from build123d import *

# Parameters (mm, degrees)
CUT_EXTRUDE_START   = 40
CUT_EXTRUDE_1_DEPTH = 15
SKETCH_3_R          = 2.5
EXTRUDE_1_DEPTH     = 3
FILLET_1_R          = 1


with BuildPart() as part:
    # 草图1 → 旋转1 (revolve)
    with BuildSketch(Plane.XY, mode=Mode.PRIVATE) as revolve_1_sk:
        with BuildLine():
            Line((0, 0), (38, 0))
            Line((38, 0), (38, 15))
            Line((38, 15), (35, 15))
            Line((35, 15), (35, 17))
            Line((35, 17), (38, 17))
            Line((38, 17), (38, 21))
            ThreePointArc((38, 21), (32.142135624, 35.142135624), (18, 41))
            Line((18, 41), (0, 41))
            Line((0, 41), (0, 0))
        make_face()
    revolve(revolve_1_sk.sketch.rotate(Axis((0, 0, 0), (0, 1, 0)), 90), axis=Axis((0, 0, 0), (0, 1, 0)))

    # 草图2 → 切除-拉伸1 (cut)
    with BuildSketch(Plane.XY.offset(CUT_EXTRUDE_START)):
        with BuildLine():
            Line((-20, 34), (20, 34))
            ThreePointArc((20, 34), (24, 30), (20, 26))
            Line((20, 26), (-20, 26))
            ThreePointArc((-20, 26), (-24, 30), (-20, 34))
        make_face()
    extrude(amount=-CUT_EXTRUDE_1_DEPTH, mode=Mode.SUBTRACT)

    # 草图3 → 凸台-拉伸1 (add)
    with BuildSketch(Plane.XY.offset(25)):
        with Locations((-20, 30)):
            Circle(SKETCH_3_R)
        with Locations((20, 30)):
            Circle(SKETCH_3_R)
    extrude(amount=EXTRUDE_1_DEPTH)

    # 圆角1
    fillet_1_edges = [part.edges().sort_by_distance(p)[0] for p in [
        (-22.5, 30, 28),
    ]]
    fillet(fillet_1_edges, radius=FILLET_1_R)


solid = part.part
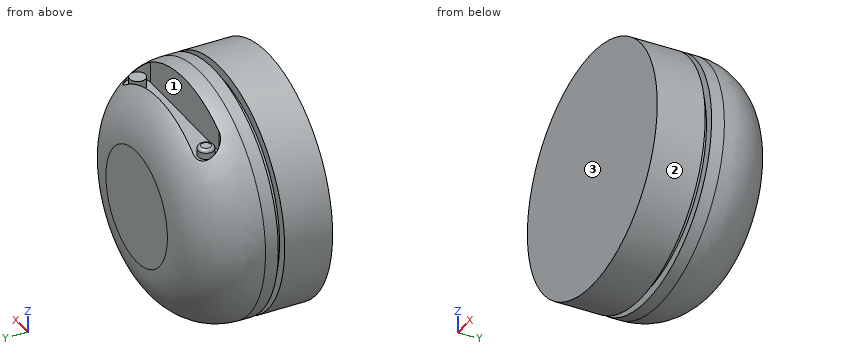
Can you work these out from the model? Positions are in its coordinate system, mm. Face numbers are marked on the shaded views. Round coordinates to 2 decimals unless told otherwise and drop trailing zeros. Write item = value, one per line. Start each with the question number.
(1) If I drill on probe 1 along Y at (x, z) = (-14, 28); probe 2 along Y at (x, z) = (15.5, -33); probe 3 along Y at (x, z) = (13, -26.5), over which ranges is the centre line in solid material (lowest first)? Write a range as [from, to].
(2) If we mould it in two halves opening along X, with no side actions, what happens to the marked faces 1, 2 and 3? For each: released by +X, released by -X, zero draft, split by the parting line, or undercut.
(3) For P1, Ø1.5, axis at x = 20, y = 30, coming from the +Z side; P2, Ø4, axis at y = 8.5, z = -2.5, coming from the +X side; P3, Ø12, axis at x = 24.5, z = -6.5, coming from the +Y side; P4, Ø2.5, axis at x = -2, z = 28.5, coming from the -Y side, each with a flat end and sliding along its axis, tell me the tip position at first contact or that it passes through.
Ans:
q1.probe_1 = [0, 26], [34, 35.93]
q1.probe_2 = [0, 15], [17, 28.7]
q1.probe_3 = [0, 37.35]
q2.face_1 = undercut
q2.face_2 = split by the parting line
q2.face_3 = zero draft
q3.P1 = 28
q3.P2 = 38
q3.P3 = 40.95
q3.P4 = 0
